from build123d import *

# Parameters (mm, degrees)
SKETCH1_W                                        = 95
SKETCH1_H                                        = 30
BOSS_EXTRUDE1_DEPTH                              = 5
CBORE_FOR_M2_HEX_HEAD_MACHINE_SCREW1_D           = 2.4
CBORE_FOR_M2_HEX_HEAD_MACHINE_SCREW1_CBORE_D     = 6.38
CBORE_FOR_M2_HEX_HEAD_MACHINE_SCREW1_CBORE_DEPTH = 1.6
M3X0_5_TAPPED_HOLE1_D                            = 2.5
M3X0_5_TAPPED_HOLE1_DEPTH                        = 3
M3X0_5_TAPPED_HOLE1_TIP                          = 0.751075774


with BuildPart() as part:
    # Sketch1 → Boss-Extrude1 (new body)
    with BuildSketch(Plane.XY):
        Rectangle(SKETCH1_W, SKETCH1_H)
    extrude(amount=BOSS_EXTRUDE1_DEPTH)

    # CBORE for M2 Hex Head Machine Screw1 (through all)
    with Locations(Plane.XY.offset(5)):
        with Locations((-42.5, 10), (-42.5, -10), (42.5, -10), (42.5, 10)):
            CounterBoreHole(CBORE_FOR_M2_HEX_HEAD_MACHINE_SCREW1_D / 2, CBORE_FOR_M2_HEX_HEAD_MACHINE_SCREW1_CBORE_D / 2, CBORE_FOR_M2_HEX_HEAD_MACHINE_SCREW1_CBORE_DEPTH)

    # M3x0.5 Tapped Hole1
    with Locations(Plane(origin=(0, 15, 0), x_dir=(1, 0, 0), z_dir=(0, 1, 0))):
        with Locations((34.061922087, -2.5), (-34.061922087, -2.5)):
            Hole(M3X0_5_TAPPED_HOLE1_D / 2, depth=M3X0_5_TAPPED_HOLE1_DEPTH)
            with Locations((0, 0, -(M3X0_5_TAPPED_HOLE1_DEPTH + M3X0_5_TAPPED_HOLE1_TIP / 2))):  # 118° drill point
                Cone(0, M3X0_5_TAPPED_HOLE1_D / 2, M3X0_5_TAPPED_HOLE1_TIP, mode=Mode.SUBTRACT)


solid = part.part
Could you check a few things on this model? Use its own coordinates, in mm. A direction names the side the tool comes from. Give positions to 0.01 mm unless a question says otherwise; leave off trailing zeros. Order: outer loops, then holes, each group sorted by start corner. A loop starts at its lowest first (then second) coordinate and runs counter-clockwise, first axis right, second up. Notation, with made-up numbers: (58, 56) -> (71, 56) arc R32 ccw to (71, 94) -> close; hole circle Ø1 at (86, -22). An arc over 180 degrees is marked (long way). Return JSON: item names as keys, results as strings.
1. I need wall thicknesses on line 1 (Y direction, x = -42.5, z = 1.6); line 2 (Y direction, x = -42.5, z = 4.3); line 3 (X direction, y = 12, z = 3.05). Which ranges of each line are inside material? Lowest first, please. Write a range as from..to.
Answer list:
{"line 1": "y = -15..-11.2, -8.8..8.8, 11.2..15", "line 2": "y = -15..-13.19, -6.81..6.81, 13.19..15", "line 3": "x = -47.5..-35.18, -32.94..32.94, 35.18..47.5"}
2. For pin 1 Ø3 at (x, y) = (-43.5, -9.5) entering from +Z, with a flat end and sliding along its axis, tell me the tip position at first contact or that it passes through.
Answer list:
{"pin 1": "stops at z = 3.4"}
3. Imagine slicing it at B-B on y = -10. List the corners of the cut face in (x, z) for me.
Answer list:
{"outline": "(-47.5, 0) -> (-43.7, 0) -> (-43.7, 3.4) -> (-45.69, 3.4) -> (-45.69, 5) -> (-47.5, 5) -> close; (-41.3, 0) -> (41.3, 0) -> (41.3, 3.4) -> (39.31, 3.4) -> (39.31, 5) -> (-39.31, 5) -> (-39.31, 3.4) -> (-41.3, 3.4) -> close; (43.7, 0) -> (47.5, 0) -> (47.5, 5) -> (45.69, 5) -> (45.69, 3.4) -> (43.7, 3.4) -> close"}
4. On a 3-axis mill with a long thin cutter (end or side, diameter ignored), from which of +Z, -Z, +X, -X, +Y, -Y can I reach the whole of each face in a straight line? I mean faces 1 (the cylindrical face through (39.313, 10.14, 4.211)), 2 (the cylindrical face through (-32.813, 13.479, 2.445)), 3 (the cylindrical face through (41.39, 9.54, 1.68)). Say none if no direction works.
Answer list:
{"face 1": "+Z", "face 2": "+Y", "face 3": "+Z, -Z"}
5. Imagine slicing it at A-A on x = 42.5. List the corners of the cut face in (y, z) for me.
Answer list:
{"outline": "(-15, 0) -> (-11.2, 0) -> (-11.2, 3.4) -> (-13.19, 3.4) -> (-13.19, 5) -> (-15, 5) -> close; (-8.8, 0) -> (8.8, 0) -> (8.8, 3.4) -> (6.81, 3.4) -> (6.81, 5) -> (-6.81, 5) -> (-6.81, 3.4) -> (-8.8, 3.4) -> close; (11.2, 0) -> (15, 0) -> (15, 5) -> (13.19, 5) -> (13.19, 3.4) -> (11.2, 3.4) -> close"}
6. Thinking about a two-plate mould opening in Y: for faces 4 (the flat face through (-42.5, -11.4, 3.4)), 5 (the flat face through (-47.5, 0, 2)), 6 (the flat face through (-1, -15, 2)), which applies, pulls with the +Y half, pulls with the -Y half, needs draft (parallel to the pull), parting line crosses it, or undercut?
Answer list:
{"face 4": "undercut", "face 5": "needs draft", "face 6": "pulls with the -Y half"}
